The listing builds one solid part. Answer for the finished solid, in the listing's coordinates (mm). Face numbers are marked on the shaded views. A direction names the side the tool comes from. Round coordinates to 2 decimals unless told otherwise and drop trailing zeros. Loops run counter-clockwise (first coordinate to the right, second up) from the corner with the lowest first, then second, coordinate; pieces in that order, holes last. Notation, with made-up numbers: M -17,67 L 20,67 A27 ccw 20,89 Z; hole C 39.5,56.25 d4. An arc over 180 degrees is marked long. Answer as a JSON object with one key per item and string values.
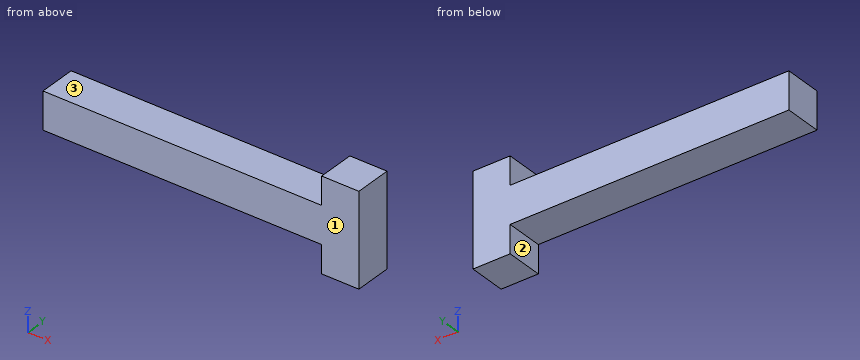
```python
from build123d import *

# Parameters (mm, degrees)
SKETCH1_W           = 15
SKETCH1_H           = 2
BOSS_EXTRUDE1_DEPTH = 2


with BuildPart() as part:
    # Sketch1 → Boss-Extrude1 (new body)
    with BuildSketch(Plane(origin=(0, 0, 0), x_dir=(1, 0, 0), z_dir=(0, 1, 0))):
        Rectangle(SKETCH1_W, SKETCH1_H)
        Polygon((7.5, 1), (7.5, -1), (7.5, -2.5), (9.5, -2.5), (9.5, 2.5), (7.5, 2.5), align=None)
    extrude(amount=BOSS_EXTRUDE1_DEPTH)


solid = part.part
```
Item 1: Flat-ended cylindrical pins translate along their axes: P1, Ø1, axis at x = 1.5, y = 1.5, coming from the -Z side; P2, Ø1.2, axis at y = 1, z = -2, coming from the -X side. Find the tip coordinate at first contact, or state that the pin passes through.
Values follow:
{"P1": "z = -1", "P2": "x = 7.5"}
Item 2: The part is cut by section B-B (z = -1.3). Give the vertices of the cut face in (x, y), then the cut area to 3 significant figures.
Values follow:
{"outline": "M 7.5,0 L 9.5,0 L 9.5,2 L 7.5,2 Z", "area": "4.00 mm^2"}
Item 3: The part is cut by section C-C (x = 0.75). Give the vertices of the cut face in (y, z), then the cut area to 3 significant figures.
Values follow:
{"outline": "M 0,-1 L 2,-1 L 2,1 L 0,1 Z", "area": "4.00 mm^2"}
Item 4: Which of the six approach directions +Z, -Z, +X, -X, +Y, -Y give full straight-line access (tool end or side, diameter ignored) to the marked faces 1, 2 and 3?
Values follow:
{"face 1": "+Z, -Z, +X, -X, -Y", "face 2": "-Z, -X, +Y, -Y", "face 3": "+Z, -X, +Y, -Y"}
Item 5: Straight lines are drawn through the part: line 1 (Z direction, x = 4, y = 0.3); line 2 (X direction, y = 0.35, z = 1.8). For each, find the intervals that lie inside material, in ascending order.
Values follow:
{"line 1": "-1 to 1", "line 2": "7.5 to 9.5"}
Item 6: The part is cut by section A-A (y = 0.55). Give the vertices of the cut face in (x, z).
Values follow:
{"outline": "M -7.5,-1 L 7.5,-1 L 7.5,-2.5 L 9.5,-2.5 L 9.5,2.5 L 7.5,2.5 L 7.5,1 L -7.5,1 Z"}
